Autodesk Inventor part; units mm, degrees
ref_plane "YZ Plane" through (0, 0, 0) normal (1, 0, 0) x (0, 1, 0)
ref_plane "XZ Plane" through (0, 0, 0) normal (0, 1, 0) x (-1, 0, 0)
ref_plane "XY Plane" through (0, 0, 0) normal (0, 0, 1) x (1, 0, 0)
sketch "スケッチ1" plane through (0, 0, 0) normal (0, 0, 1) x (1, 0, 0)
  circle A0 centre (0, 0) radius 1.5
  dimension "d0" = 3
extrude "押し出し1" add sketch "スケッチ1" along normal blind 24
sketch "スケッチ2" plane through (0, 0, 24) normal (0, 0, 1) x (1, 0, 0)
  circle A0 centre (0, 0) radius 1.5
  circle A1 centre (0, 0) radius 3
  dimension "d3" = 6
extrude "押し出し2" add sketch "スケッチ2" along normal blind 2 contours A0 | A1
fillet "フィレット1" radius 2 1 edges at (-3, 0, 26)
properties part number "M3ボタンボルト15" material "鋼、高強度、低合金"
CAD build for the part. Positions are in the model's coordinates, mm. A direction names the side the tool comes from. Round coordinates to 2 decimals unless told otherwise and drop trailing zeros. Order: outer loops, then holes, each group sorted by start corner. A loop starts at its lowest first (then second) coordinate and runs counter-clockwise, first axis right, second up. Notation, with made-up numbers: (-25.5, -14.75) - (24.5, -14.75) arc R17 cw to (24.5, -7.75) - close; hole circle Ø4 at (34, 60.25). An arc over 180 degrees is marked (long way). Use CSV: the item, a comma, the result in double quotes. Start each with the question number.
1) Pin check, flat tips, straight feed: pin 1 Ø2 at (y, z) = (2, 3) entering from -X; pin 2 Ø1.5 at (x, y) = (-1, -0.5) entering from +Z; pin 3 Ø2 at (x, z) = (2, 4.5) entering from +Y. Stop position of each tip, or through.
2) Wall check: L1, parallel to Y at x = 0, z = 8.5; L2, parallel to Z at x = -1.5, y = -1.75; L3, parallel to Z at x = -1, y = 0.5. Give the ranges that are in metal, low to high. Write a range as [from, to].
3) Saw through at A-A (z = 14.25). List the corners of the cut face in (x, y), and give its area (3 significant figures).
4) Tool access for faces 1 (the flat face through (0, 0, 0)), 2 (the cylindrical face through (-1.5, -0.07, 11.83)): list every direction of +Z, -Z, +X, -X, +Y, -Y with a clear straight run to the whole face (end or side of a thin tool).
Values follow:
1,pin 1,"stops at x = -1.12"
1,pin 2,"stops at z = 26"
1,pin 3,"stops at y = 1.12"
2,L1,"y = [-1.5, 1.5]"
2,L2,"z = [24, 25.52]"
2,L3,"z = [0, 26]"
3,outline,"circle Ø3 at (0, 0)"
3,area,"7.07 mm2"
4,face 1,"-Z, +X, -X, +Y, -Y"
4,face 2,"-Z"
